Input: part model. Units: mm. Frame: model coordinates. A direction names the side the tool comes from. Coordinates: 2 decimals unless noted, no trailing zeros. Write each loop counter-clockwise with the first axis right and the second up, starting at its lowest first coordinate (ties: lowest second). Pieces come first, ordered by that corner, then holes. Notation, with made-up numbers: M -25,52.25 L -14,52.25 A6 ccw -14,62.25 Z; hole C 33,15 d2. An arc over 180 degrees is marked long. Write each question's results on one line, items separated by ' | '. Start each with the question number.
1. First-contact query: pin 1 (1 mm diameter, centred on y = -5, z = 8.5, fed in from -X); pin 2 (12 mm diameter, centred on y = -13.5, z = 0, fed in from +X) (3 decimals); pin 3 (1.9 mm diameter, centred on y = 2, z = 10.5, fed in from +X). Flat tips, straight axial feed; report the tip coordinate or a pass-through.
2. Section query B-B, the plane z = 7.5. Output: boundary loops of the cut face in (x, y).
3. Set-up query: faces 1 (the cylindrical face through (-1.932, -12.522, 7.663)), 2 (the cylindrical face through (-10.795, 2.692, -2.545)), 3 (the cylindrical face through (13.952, 3.21, 14.128)). Return all of +Z, -Z, +X, -X, +Y, -Y with unobstructed straight access to the full face (end or side cutting, diameter ignored); none if empty.
4. Pull-direction query (X, two-part tool) for faces 4 (the flat face through (6.223, 3, -2)), 5 (the cylindrical face through (-0.046, 3.21, 14.128)), 6 (the cylindrical face through (10.668, 2.692, -2.545)), 7 (the flat face through (-15.24, 3, 13)); classes: +X half, -X half, draft (parallel to the pull), parting line (faces both ways), or undercut.
5. Ray query, probe 1 along X at (y, z) = (4.5, -4.75); probe 2 along Y at (x, z) = (-4, 11); probe 3 along X at (y, z) = (1.5, 6). Return the intervals inside material, ascending.
```python
from build123d import *

# Parameters (mm, degrees)
FINGERBASE_DEPTH         = 6.35
BOSS_EXTRUDE1_DEPTH      = 2.54
BOSS_EXTRUDE1_DEPTH_BACK = 27.94
SKETCH2_R                = 0.79375
SKETCH3_R                = 3.175
BOSS_EXTRUDE2_DEPTH      = 25.4


with BuildPart() as part:
    # Sketch1 → FingerBase (new body)
    with BuildSketch(Plane(origin=(0, 0, 0), x_dir=(1, 0, 0), z_dir=(0, 1, 0))):
        Polygon((-6.223, 6.223), (6.223, 6.223), (6.223, -1.7145), (12.7, -1.7145), (12.7, -16.51), (3.302, -16.51), (3.302, -8.5725), (-3.302, -8.5725), (-3.302, -16.51), (-12.7, -16.51), (-12.7, -1.7145), (-6.223, -1.7145), align=None)
    extrude(amount=FINGERBASE_DEPTH)

    # Sketch2 → Boss-Extrude1 (add, two sides: drawn at the far end of the back side and taken through both)
    with BuildSketch(Plane(origin=(12.7, 0, 0), x_dir=(0, 0, -1), z_dir=(1, 0, 0)).offset(-BOSS_EXTRUDE1_DEPTH_BACK)):
        with Locations((-13.335, 3.175)):
            Circle(SKETCH2_R)
        with Locations((3.175, 3.175)):
            Circle(SKETCH2_R)
    extrude(amount=BOSS_EXTRUDE1_DEPTH + BOSS_EXTRUDE1_DEPTH_BACK)

    # Sketch3 → Boss-Extrude2 (add)
    with BuildSketch(Plane.XZ):
        with Locations(Location((0, 5.1435, 0), (0, 0, 270))):
            Circle(SKETCH3_R)
    extrude(amount=BOSS_EXTRUDE2_DEPTH)


solid = part.part
```
Answer:
1) pin 1: x = -1.39 | pin 2: x = 3.175 | pin 3: x = 12.7
2) outline: M -12.7,0 L -2.13,0 L -2.13,-25.4 L 2.13,-25.4 L 2.13,0 L 12.7,0 L 12.7,6.35 L -12.7,6.35 Z
3) face 1: -Y | face 2: -X | face 3: +X
4) face 4: +X half | face 5: undercut | face 6: draft | face 7: -X half
5) probe 1: -6.22 to 6.22 | probe 2: 0 to 6.35 | probe 3: -12.7 to 12.7
